For this review, use the dimensioned drawing (mm, ordinates from the lowest corner) and the shaded views. Coordinates: 2 decimals unless noted, no trailing zeros. Loops run counter-clockwise (first coordinate to the right, second up) from the corner with the lowest first, then second, coordinate; pieces in that order, holes last. Notation, with made-up numbers: (-13, 15) - (27, 15) arc R8 ccw to (27, 21) - close; hole circle Ø10 at (82, -17.75). An arc over 180 degrees is marked (long way). Answer in a Markdown table with one row per item. Add a question column.
(1) We need section C-C, the plane y = 52. Write out the cut boundary in (x, z).
(2) We need section A-A, the plane z = 29.5. Write out the cut boundary in (x, y), plus the area to 3 significant figures.
(3) To check wall thickness, follow L1, parallel to Z at x = 4.05, y = 53.5; L2, parallel to Y at x = 3.55, z = 12.5; L3, parallel to Z at x = 4.25, y = 15 (1 decimal). State the ranges of each line that lie inside material, in increasing order. Write a range as [from, to].
(4) We need section B-B, the plane x = 1.5. Write out the cut boundary in (y, z), plus the area to 3 significant figures.
(5) We need section D-D, the plane z = 17. Write out the cut boundary in (x, y).
(6) Clearance check with flat-ended pins moving along their axes: pin 1 (1 mm diameter, centred on y = 39, z = 22, fed in from -X); pin 2 (3 mm diameter, centred on y = 49.64, z = 29.5, fed in from -X). State where each tip first meets the part, or that it passes through.
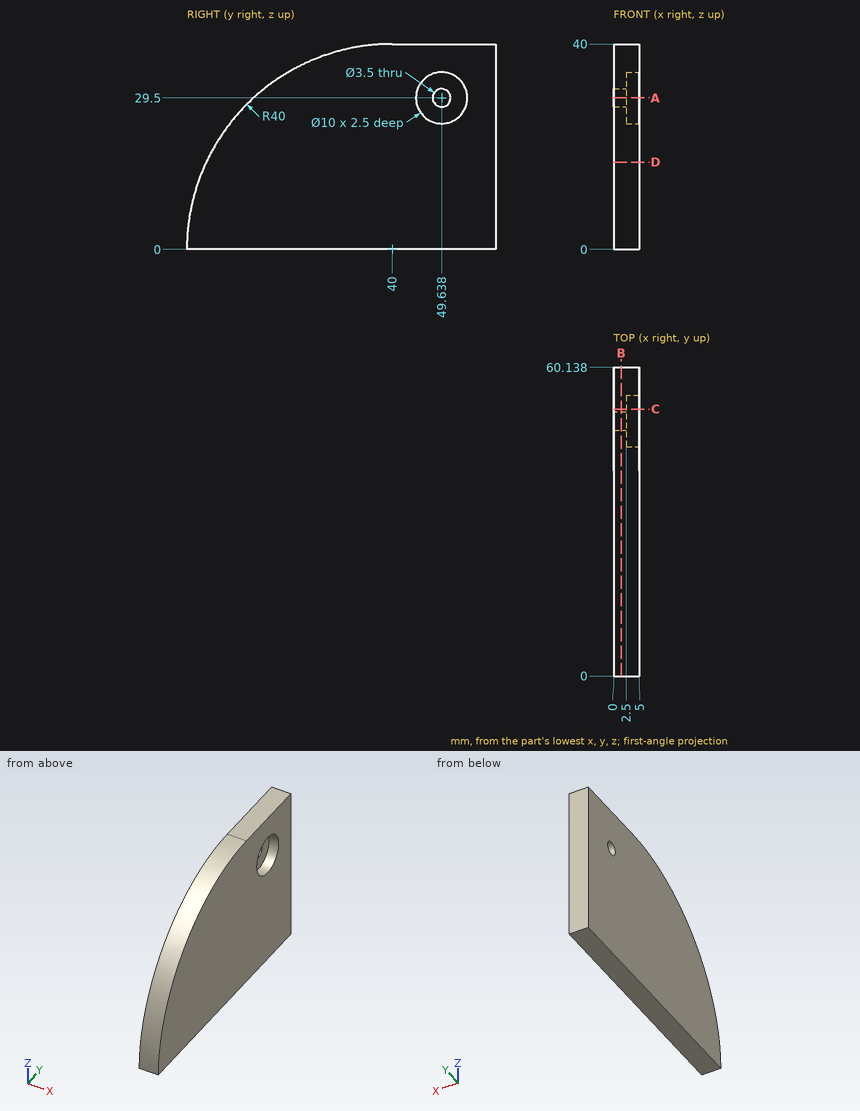
Responses:
| question | item | result |
|---|---|---|
| 1 | outline | (0, 0) - (5, 0) - (5, 25.09) - (2.5, 25.09) - (2.5, 33.91) - (5, 33.91) - (5, 40) - (0, 40) - close |
| 2 | outline | (0, 12.99) - (5, 12.99) - (5, 44.64) - (2.5, 44.64) - (2.5, 47.89) - (0, 47.89) - close; (0, 51.39) - (2.5, 51.39) - (2.5, 54.64) - (5, 54.64) - (5, 60.14) - (0, 60.14) - close |
| 2 | area | 202 mm2 |
| 3 | L1 | z = [0, 26.32], [32.68, 40] |
| 3 | L2 | y = [2, 60.14] |
| 3 | L3 | z = [0, 31.2] |
| 4 | outline | (0, 0) - (60.14, 0) - (60.14, 40) - (40, 40) arc R40 ccw to start; hole circle Ø3.5 at (49.64, 29.5) |
| 4 | area | 2,050 mm2 |
| 5 | outline | (0, 3.79) - (5, 3.79) - (5, 60.14) - (0, 60.14) - close |
| 6 | pin 1 | stops at x = 0 |
| 6 | pin 2 | passes through |
